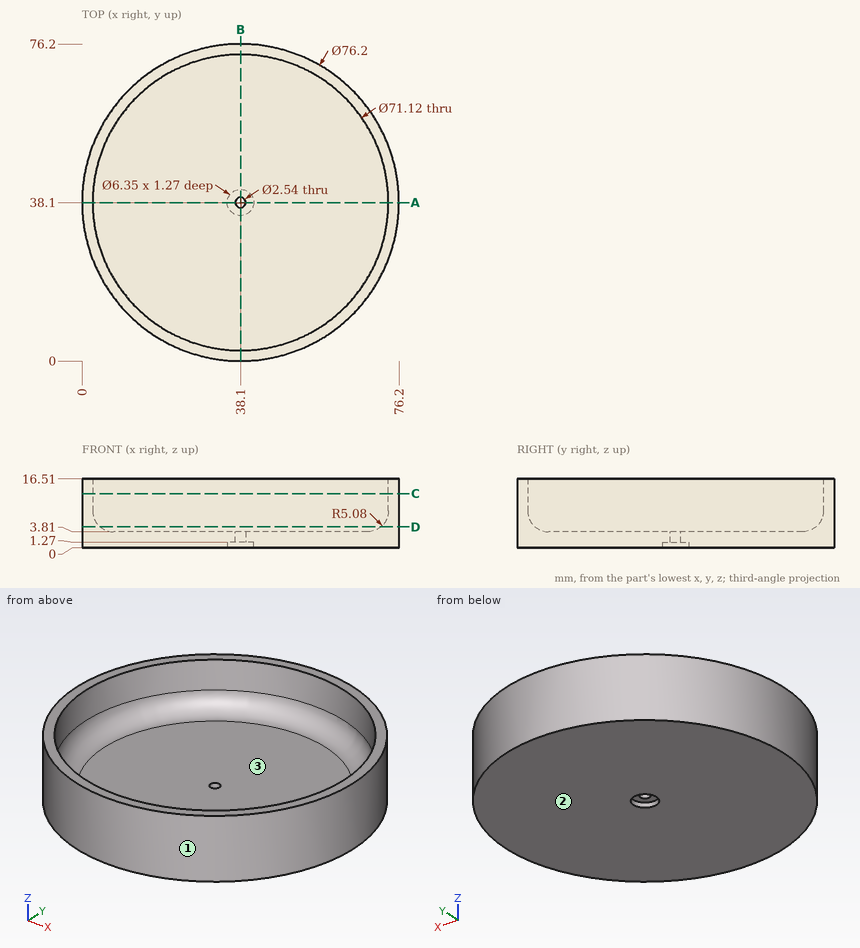
Check sheet for the drawn part. Datum: minimum x, y, z corner. Units: mm. Coordinates: 2 decimals unless noted, no trailing zeros. Loops run counter-clockwise (first coordinate to the right, second up) from the corner with the lowest first, then second, coordinate; pieces in that order, holes last. Notation, with made-up numbers: (-12, 60.25) -> (17, 60.25) arc R8 cw to (17, 75.25) -> close; hole circle Ø2 at (-31.75, 8.5). An arc over 180 degrees is marked (long way). Write each question's results on one line, items separated by ' | '.
Item 1: Section check C-C, the plane z = 13. Enter the section's corners in (x, y).
Found:
outline: circle Ø76.2 at (38.1, 38.1); hole circle Ø71.12 at (38.1, 38.1)
Item 2: Gauge pin test, flat ends, axial feed: pin 1 (2 mm diameter, centred on x = 59, y = 23.5, fed in from -Z); pin 2 (10 mm diameter, centred on x = 38.1, y = 38.1, fed in from +Z); pin 3 (5 mm diameter, centred on x = 44, z = 13, fed in from -Y); pin 4 (2 mm diameter, centred on x = 19, z = 10.5, fed in from -Y). Record the tip position at first contact, or that the pin passes through.
Found:
pin 1: stops at z = 0 | pin 2: stops at z = 3.81 | pin 3: stops at y = 0.15 | pin 4: stops at y = 4.57
Item 3: Section check A-A, the plane y = 38.1. Enter the section's corners in (x, z) (3 decimals).
Found:
outline: (0, 0) -> (34.925, 0) -> (34.925, 1.27) -> (36.83, 1.27) -> (36.83, 3.81) -> (7.62, 3.81) arc R5.08 cw to (2.54, 8.89) -> (2.54, 16.51) -> (0, 16.51) -> close; (39.37, 1.27) -> (41.275, 1.27) -> (41.275, 0) -> (76.2, 0) -> (76.2, 16.51) -> (73.66, 16.51) -> (73.66, 8.89) arc R5.08 cw to (68.58, 3.81) -> (39.37, 3.81) -> close
Item 4: Mould release check, pull along Y, two halves, no side actions. Record for the marked faces 1, 2 and 3: +Y half, -Y half, draft (parallel to the pull), parting line (faces both ways), or undercut.
Found:
face 1: parting line | face 2: draft | face 3: undercut
Item 5: Material ranges on L1, parallel to X at y = 37, z = 11; L2, parallel to Y at x = 38, z = 11; L3, parallel to Y at x = 38.1, z = 0.6 (3 decimals), recorded low to high.
Found:
L1: x = 0.02 to 2.56, 73.64 to 76.18 | L2: y = 0 to 2.54, 73.66 to 76.2 | L3: y = 0 to 34.925, 41.275 to 76.2
Item 6: Section check D-D, the plane z = 5. Enter the section's corners in (x, y), plus the area to 4 significant figures.
Found:
outline: circle Ø76.2 at (38.1, 38.1); hole circle Ø67.49 at (38.1, 38.1) | area: 982.5 mm2
